Part print with two shaded views. Sizes in mm from the minimum x, y, z corner. Round coordinates to 2 decimals unless told otherwise and drop trailing zeros. Loops run counter-clockwise (first coordinate to the right, second up) from the corner with the lowest first, then second, coordinate; pieces in that order, holes last.
(1) Flat gauge pin, fed straight in: pin 1 (7 mm diameter, centred on x = 75, y = 110, fed in from +Z). Where does the tip first touch, or does it go through?
(2) Cut at A-A on x = 75. List the corners of the cut face in (y, z).
(3) Cut at B-B on y = 145. List the corners of the cut face in (x, z), then the cut area to 3 significant figures.
(4) Cut at C-C on z = 10.25. Count the separate pieces of the cut face and the enclosed holes in it, then the cut area to 3 significant figures.
(5) Probe probe 1 along Y at (x, z) = (25, 4.5); probe 2 along Y at (x, z) = (86, 7.25); probe 3 along X at (y, z) = (14, 3). List the from-to ranges inside material, lowest first.
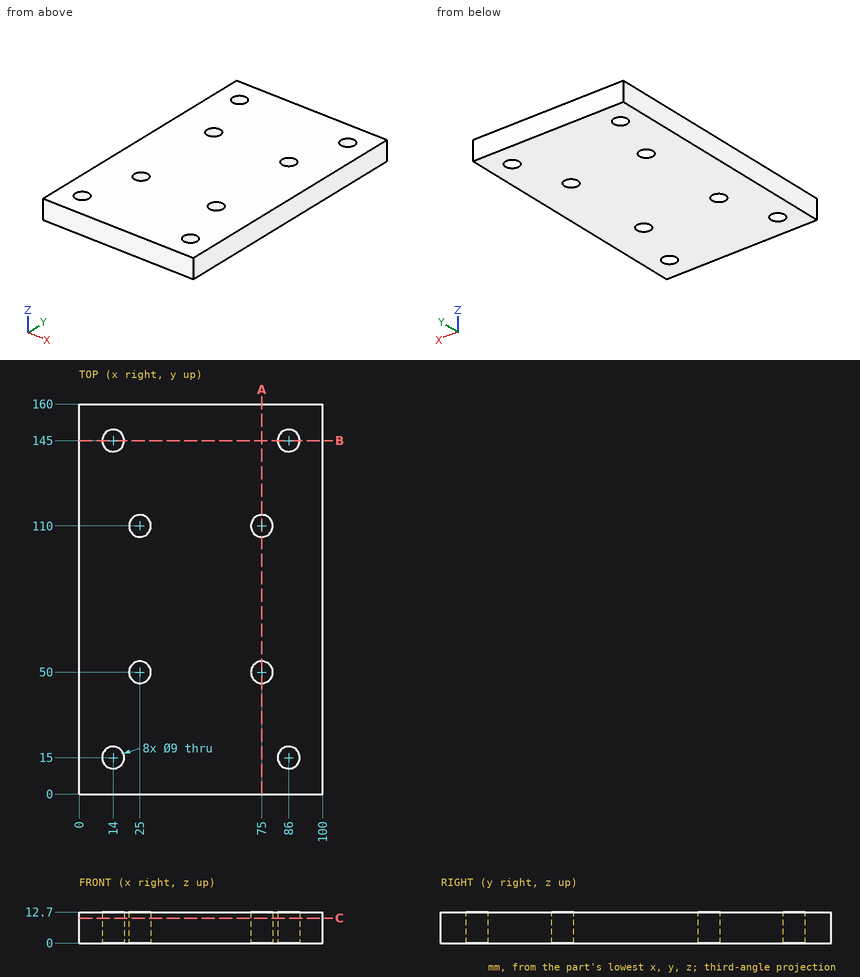
Final values:
1. pin 1: passes through
2. outline: (0, 0) - (45.5, 0) - (45.5, 12.7) - (0, 12.7) - close; (54.5, 0) - (105.5, 0) - (105.5, 12.7) - (54.5, 12.7) - close; (114.5, 0) - (160, 0) - (160, 12.7) - (114.5, 12.7) - close
3. outline: (0, 0) - (9.5, 0) - (9.5, 12.7) - (0, 12.7) - close; (18.5, 0) - (81.5, 0) - (81.5, 12.7) - (18.5, 12.7) - close; (90.5, 0) - (100, 0) - (100, 12.7) - (90.5, 12.7) - close
3. area: 1,040 mm2
4. separate pieces: 1
4. enclosed holes: 8
4. area: 15,500 mm2
5. probe 1: y = 0 to 45.5, 54.5 to 105.5, 114.5 to 160
5. probe 2: y = 0 to 10.5, 19.5 to 140.5, 149.5 to 160
5. probe 3: x = 0 to 9.61, 18.39 to 81.61, 90.39 to 100
